```python
from build123d import *

# Parameters (mm, degrees)
F1_DEPTH = 25
F2_R     = 14.726703
F3_R     = 26.314928


with BuildPart() as f1:
    # F0 (on Top) → F1 (new body)
    with BuildSketch(Plane.XY):
        Polygon((148.460492, 13.362525), (-151.539508, 13.362525), (-151.539508, -37.299059), (-141.539508, -37.299059), (-141.539508, 3.362525), (138.460492, 3.362525), (138.460492, -37.299059), (148.460492, -37.299059), align=None)
    extrude(amount=F1_DEPTH)

    # F2
    f2_edges = [f1.edges().sort_by_distance(p)[0] for p in [
        (-141.539508, 3.362525, 12.5),
        (138.460492, 3.362525, 12.5),
    ]]
    fillet(f2_edges, radius=F2_R)

    # F3
    f3_edges = [f1.edges().sort_by_distance(p)[0] for p in [
        (-151.539508, 13.362525, 12.5),
        (148.460492, 13.362525, 12.5),
    ]]
    fillet(f3_edges, radius=F3_R)


solid = f1.part
```
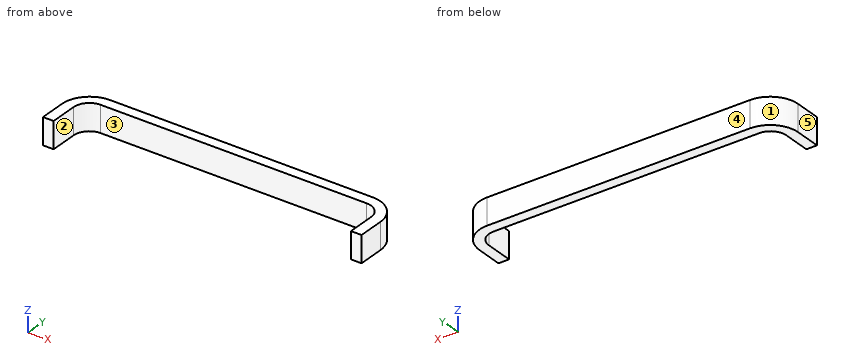
Source: CAD feature listing. Evaluate the final solid. Frame: model axes, mm. Face numbers are marked on the shaded views. A direction names the side the tool comes from. Round coordinates to 2 decimals unless told otherwise and drop trailing zeros. Loops run counter-clockwise (first coordinate to the right, second up) from the corner with the lowest first, then second, coordinate; pieces in that order, holes last. Notation, with made-up numbers: M 47,75 L 104,75 A30 cw 104,97 Z; hole C 20,-22 d5. An arc over 180 degrees is marked long. Use a Markdown table: item, result. Add a question column.
1. Section query C-C on y = -8. Return the cut outline in (x, z), then the cut area to 3 significant figures.
2. Line query: line 1 (X direction, y = -19, z = 21); line 2 (Y direction, x = 98.5, z = 5.75); line 3 (Y direction, x = 123.5, z = 8). Output: solid intervals per line, ascending.
3. Section query D-D on x = 47.5. Return the cut outline in (y, z).
4. Mould query, pull axis X, two halves, no side actions, for the marked faces 3, 4 and 5. Classes: pulls with the +X half, pulls with the -X half, needs draft (parallel to the pull), parting line crosses it, or undercut.
5. Contact query for flat-ended pins moving along their axis: P1, Ø1, axis at x = 35, z = 18.5, coming from the -Y side; P2, Ø1, axis at y = -3, z = 8, coming from the +X side; P3, Ø4, axis at y = 0.5, z = 7, coming from the +X side. Output: stop coordinate, or through.
6. Reachability of the marked faces 1 and 2 from +Z, -Z, +X, -X, +Y, -Y: full face, straight path, thin tool, end or side. Return the list, or none.
7. Section query A-A on y = -33. Return the cut outline in (x, z).
8. Section query B-B on z = 19.25. Return the cut outline in (x, y).
Reported:
| question | item | result |
|---|---|---|
| 1 | outline | M -151.07,0 L -141.15,0 L -141.15,25 L -151.07,25 Z; M 138.07,0 L 147.99,0 L 147.99,25 L 138.07,25 Z |
| 1 | area | 496 mm² |
| 2 | line 1 | x = -151.54 to -141.54, 138.46 to 148.46 |
| 2 | line 2 | y = 3.36 to 13.36 |
| 2 | line 3 | y = 3.36 to 13.33 |
| 3 | outline | M 3.36,0 L 13.36,0 L 13.36,25 L 3.36,25 Z |
| 4 | face 3 | undercut |
| 4 | face 4 | needs draft |
| 4 | face 5 | pulls with the -X half |
| 5 | P1 | stops at y = 3.36 |
| 5 | P2 | stops at x = 146.7 |
| 5 | P3 | stops at x = 145.84 |
| 6 | face 1 | +Z, -Z, -X, +Y |
| 6 | face 2 | +Z, -Z, -Y |
| 7 | outline | M -151.54,0 L -141.54,0 L -141.54,25 L -151.54,25 Z; M 138.46,0 L 148.46,0 L 148.46,25 L 138.46,25 Z |
| 8 | outline | M -151.54,-37.3 L -141.54,-37.3 L -141.54,-11.36 A14.73 cw -126.81,3.36 L 123.73,3.36 A14.73 cw 138.46,-11.36 L 138.46,-37.3 L 148.46,-37.3 L 148.46,-12.95 A26.31 ccw 122.15,13.36 L -125.22,13.36 A26.31 ccw -151.54,-12.95 Z |
